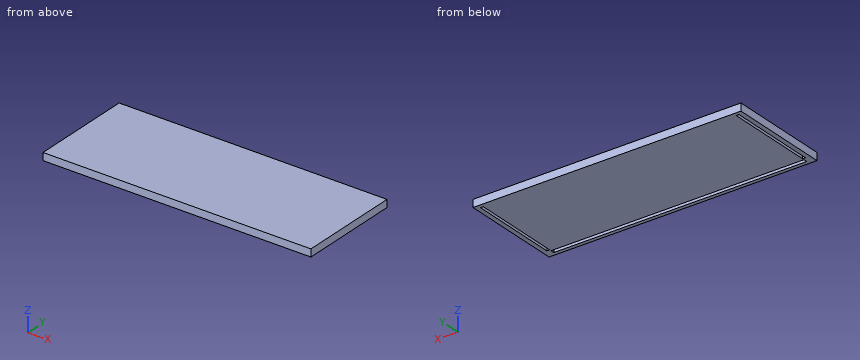
from build123d import *

# Parameters (mm, degrees)
F0_W     = 914.4
F0_H     = 349.25
F1_DEPTH = 12.7
F2_W     = 863.6
F2_H     = 12.7
F3_DEPTH = 12.7
F4_W     = 9.525
F4_H     = 304.8
F5_DEPTH = 12.7


# Not quite as in the source:
# - a feature names something its author has since deleted; it is built from what else it names


with BuildPart() as f1:
    # F0 (on Top) → F1 (new body, symmetric)
    with BuildSketch(Plane.XY):
        Rectangle(F0_W, F0_H)
    extrude(amount=F1_DEPTH, both=True)

    # F2 (on face) → F3 (cut)
    with BuildSketch(Plane(origin=(0, 0, -12.7), x_dir=(1, 0, 0), z_dir=(0, 0, -1))):
        with Locations((0, 155.575)):
            Rectangle(F2_W, F2_H)
    extrude(amount=-F3_DEPTH, mode=Mode.SUBTRACT)

    # F4 (on face) → F5 (cut)
    with BuildSketch(Plane(origin=(0, 0, -12.7), x_dir=(1, 0, 0), z_dir=(0, 0, -1))):
        with Locations((-436.5625, -9.525)):
            Rectangle(F4_W, F4_H)
        with Locations((436.5625, -9.525)):
            Rectangle(F4_W, F4_H)
    extrude(amount=-F5_DEPTH, mode=Mode.SUBTRACT)


solid = f1.part
Could you check a few things on this model? Use its own coordinates, in mm. Coordinates: 2 decimals unless noted, no trailing zeros. Order: outer loops, then holes, each group sorted by start corner. A loop starts at its lowest first (then second) coordinate and runs counter-clockwise, first axis right, second up. Notation, with made-up numbers: (40.25, -15.5) -> (51.25, -15.5) arc R15 cw to (51.25, 0.5) -> close; hole circle Ø10 at (31, 44). An arc over 180 degrees is marked (long way). One line per item, written item: value. Start each with the question number.
1) I'm going to push a flat-ended pin straight in: pin 1 (4 mm diameter, centred on x = -6, y = -153, fed in from -Z). Where does the tip first touch, or does it pass through?
2) Imagine slicing it at A-A on x = 219. List the corners of the cut face in (y, z) for me (3 decimals), plus the area to 3 significant figures.
3) If I drill on L1, parallel to X at y = 141.5, z = -3.5 (3 decimals); L2, parallel to Y at x = -137.5, z = -4.5 (3 decimals); L3, parallel to Z at x = -239, y = -153.5, over which ranges is the centre line in solid material (lowest first)? Write a range as [from, to].
Answer list:
1. pin 1: stops at z = 0
2. outline: (-174.625, -12.7) -> (-161.925, -12.7) -> (-161.925, 0) -> (-149.225, 0) -> (-149.225, -12.7) -> (174.625, -12.7) -> (174.625, 12.7) -> (-174.625, 12.7) -> close
2. area: 8,710 mm2
3. L1: x = [-457.2, -441.325], [-431.8, 431.8], [441.325, 457.2]
3. L2: y = [-174.625, -161.925], [-149.225, 174.625]
3. L3: z = [0, 12.7]
